from build123d import *

# Parameters (mm, degrees)
BOSS_EXTRUDE1_DEPTH              = 12.7
CUT_EXTRUDE1_DEPTH               = 13.7
HOLE1_D                          = 30
HOLE1_DEPTH                      = 12.7
HOLE2_D                          = 47
HOLE2_DEPTH                      = 12.7
F_39_0_0995_DIAMETER_HOLE1_D     = 2.5273
F_39_0_0995_DIAMETER_HOLE1_DEPTH = 12.7
F_4_CLEARANCE_HOLE1_D            = 3.3
F_4_CLEARANCE_HOLE1_DEPTH        = 12.7
F_2_CLEARANCE_HOLE1_D            = 2.499999999
F_2_CLEARANCE_HOLE1_DEPTH        = 12.7
F_4_CLEARANCE_HOLE2_D            = 3.3
F_4_CLEARANCE_HOLE2_DEPTH        = 10


with BuildPart() as part:
    # Sketch1 → Boss-Extrude1 (new body)
    with BuildSketch(Plane.XY.offset(12.7)):
        with BuildLine():
            Line((-30, 305), (-30, 23.323807579))
            Line((-30, 23.323807579), (-30, -23.323807579))
            ThreePointArc((-30, -23.323807579), (0, -38), (30, -23.323807579))
            Line((30, -23.323807579), (30, 23.323807579))
            Line((30, 23.323807579), (30, 305))
            ThreePointArc((30, 305), (0, 335), (-30, 305))
        make_face()
    extrude(amount=-BOSS_EXTRUDE1_DEPTH)

    # Sketch2 → Cut-Extrude1 (cut, through all)
    with BuildSketch(Plane(origin=(0, 0, 0), x_dir=(-1, 0, 0), z_dir=(0, 0, -1))):
        with BuildLine():
            Line((18.5, 74.022471071), (18.5, 84.022471071))
            ThreePointArc((18.5, 84.022471071), (0, 102.522471071), (-18.5, 84.022471071))
            Line((-18.5, 84.022471071), (-18.5, 74.022471071))
            ThreePointArc((-18.5, 74.022471071), (0, 55.522471071), (18.5, 74.022471071))
        make_face()
    extrude(amount=-CUT_EXTRUDE1_DEPTH, mode=Mode.SUBTRACT)

    # Hole1
    with Locations(Plane.XY.offset(12.7)):
        with Locations((0, 0)):
            Hole(HOLE1_D / 2, depth=HOLE1_DEPTH)

    # Hole2
    with Locations(Plane.XY.offset(12.7)):
        with Locations((0, 305)):
            Hole(HOLE2_D / 2, depth=HOLE2_DEPTH)

    # #39 (0.0995) Diameter Hole1
    with Locations(Plane.XY.offset(12.7)):
        with Locations((-26.75, 74.022471071), (-26.75, 129.511235535), (-26.75, 186.111235535), (-26.750000001, 192.911235535), (-26.750000001, 249.511235535), (-26.750000001, 305), (-3.300000001, 331.545668196), (3.299999999, 331.545668196), (26.749999999, 305), (26.749999999, 249.511235535), (26.749999999, 192.911235535), (26.75, 186.111235535), (26.75, 129.511235535), (26.75, 74.022471071), (3.4, 47.489425637), (-3.3, 47.476802874), (-23.166179551, 318.375), (-23.166179551, 291.625), (0, 278.25), (23.166179551, 291.625), (23.166179551, 318.375), (0, 331.75)):
            Hole(F_39_0_0995_DIAMETER_HOLE1_D / 2, depth=F_39_0_0995_DIAMETER_HOLE1_DEPTH)

    # #4 Clearance Hole1
    with Locations(Plane(origin=(0, 0, 0), x_dir=(-1, 0, 0), z_dir=(0, 0, -1))):
        with Locations((-25.5016, 66.772471071), (-25.5016, 91.272471071), (14.424978336, 14.424978336), (20.4, 0), (14.424978336, -14.424978336), (0, -20.4), (-14.424978336, -14.424978336), (-20.4, 0), (-14.424978336, 14.424978336), (0, 20.4), (25.5016, 66.772471071), (25.5016, 91.272471071)):
            Hole(F_4_CLEARANCE_HOLE1_D / 2, depth=F_4_CLEARANCE_HOLE1_DEPTH)

    # #2 Clearance Hole1
    with Locations(Plane(origin=(0, 0, 0), x_dir=(-1, 0, 0), z_dir=(0, 0, -1))):
        with Locations((-1.619921459, 231.265288591), (-21.578861519, 245.43367635)):
            Hole(F_2_CLEARANCE_HOLE1_D / 2, depth=F_2_CLEARANCE_HOLE1_DEPTH)

    # #4 Clearance Hole2
    with Locations(Plane(origin=(30, 0, 0), x_dir=(0, 0, -1), z_dir=(1, 0, 0))):
        with Locations((-6.35, 285.723807579), (-6.35, 133.323807579)):
            Hole(F_4_CLEARANCE_HOLE2_D / 2, depth=F_4_CLEARANCE_HOLE2_DEPTH)


solid = part.part
Geometry check sheet. Reference: the model listing, model coordinates, mm. A direction names the side the tool comes from. Give positions to 0.01 mm unless a question says otherwise; leave off trailing zeros.
1) Cross-section at A-A (z = 10.5). Give the number of separate pieces and of enclosed holes in the cut face, then the cut area to 3 significant figures.
Results are:
separate pieces: 1
enclosed holes: 39
area: 17,600 mm2
2) Draft check along X on faces 3 (the cylindrical face through (3.06, 328.3, 6.26)), 4 (the flat face through (0, 151, 12.7)), 5 (the flat face through (-30, 143, 6)), 6 (the cylindrical face through (0.66, 334.993, 6.439)). Enter one of: released by +X, released by -X, zero draft, split by the parting line, or undercut.
Results are:
face 3: undercut
face 4: zero draft
face 5: released by -X
face 6: split by the parting line
3) Material ranges on probe 1 along Y at (x, z) = (-9.5, 7.5); probe 2 along Y at (x, z) = (3.3, 3.25); probe 3 along Y at (x, z) = (-7.5, 10), recorded low to high.
Results are:
probe 1: y = -36.79 to -11.61, 11.61 to 58.15, 99.9 to 283.51, 326.49 to 333.46
probe 2: y = -37.86 to -14.63, 14.63 to 46.23, 48.75 to 55.82, 102.23 to 281.73, 328.27 to 330.28, 332.81 to 334.82
probe 3: y = -37.25 to -12.99, 12.99 to 57.11, 100.93 to 282.73, 327.27 to 334.05
4) Gauge pin test, flat ends, axial feed: pin 1 (5 mm diameter, centred on x = 12.5, z = 6.5, fed in from -Y); pin 2 (1.5 mm diameter, centred on x = 26.75, y = 192.91, fed in from +Z); pin 3 (1.5 mm diameter, centred on x = -2, z = 3.5, fed in from -Y); pin 4 (1.5 mm diameter, centred on x = 5.5, z = 8.5, fed in from -Y). Record the tip position at first contact, or that the pin passes through.
Results are:
pin 1: stops at y = -36.66
pin 2: passes through
pin 3: stops at y = -37.98
pin 4: stops at y = -37.7
5) Tool access check on faces 1 (the flat face through (-18.5, 79, 6)), 2 (the cylindrical face through (0, -38, 6)). Record the directions out of +Z, -Z, +X, -X, +Y, -Y that give a thin tool (end or side, any length) a straight path to the whole face; none if there is none.
Results are:
face 1: +Z, -Z
face 2: +Z, -Z, -Y
